The listing builds one solid part. Answer for the finished solid, in the listing's coordinates (mm). A direction names the side the tool comes from. Give positions to 0.01 mm unless a question says otherwise; leave off trailing zeros. Loops run counter-clockwise (first coordinate to the right, second up) from the corner with the lowest first, then second, coordinate; pieces in that order, holes last. Notation, with made-up numbers: (37.5, 54.5) - (49.5, 54.5) arc R13 cw to (49.5, 58.5) - close; hole circle Ø11 at (22.25, 63). An arc over 180 degrees is marked (long way). Write each question's results on one line, items separated by ' | '.
Autodesk Inventor part; units mm, degrees
ref_plane "YZ Plane" through (0, 0, 0) normal (1, 0, 0) x (0, 1, 0)
ref_plane "XZ Plane" through (0, 0, 0) normal (0, 1, 0) x (-1, 0, 0)
ref_plane "XY Plane" through (0, 0, 0) normal (0, 0, 1) x (1, 0, 0)
sketch "スケッチ1" plane through (0, 0, 0) normal (0, 0, 1) x (1, 0, 0)
  line L0 (-20, -10) -> (20, -10)
  line L1 (20, -10) -> (20, 10)
  line L2 (20, 10) -> (-20, 10)
  line L3 (-20, 10) -> (-20, -10)
  line L4 (-20, -10) -> (20, 10) construction
  line L5 (20, -10) -> (-20, 10) construction
  point P0 (0, 0)
  dimension "d0" = 40
  dimension "d1" = 20
extrude "押し出し1" add sketch "スケッチ1" along normal blind 3
sketch "スケッチ2" plane through (0, 0, 3) normal (0, 0, 1) x (1, 0, 0)
  line L0 (-16, -6) -> (16, -6) construction
  line L1 (16, -6) -> (16, 6) construction
  line L2 (16, 6) -> (-16, 6) construction
  line L3 (-16, 6) -> (-16, -6) construction
  line L4 (-16, -6) -> (16, 6) construction
  line L5 (16, -6) -> (-16, 6) construction
  point P0 (0, 0)
  dimension "d4" = 32
  dimension "d5" = 12
hole "穴1" at (-16, 6, 3) at (-16, -6, 3) at (16, -6, 3) at (16, 6, 3) direction (0, 0, -1) diameter 3.5 depth 8
sketch "スケッチ3" plane through (0, 0, 3) normal (0, 0, 1) x (1, 0, 0)
  circle A0 centre (-16, 6) radius 1.75
  line L0 (-16, 2.7668) -> (-18.8, 4.3834)
  line L1 (-18.8, 4.3834) -> (-18.8, 7.6166)
  line L2 (-18.8, 7.6166) -> (-16, 9.2332)
  line L3 (-16, 9.2332) -> (-13.2, 7.6166)
  line L4 (-13.2, 7.6166) -> (-13.2, 4.3834)
  line L5 (-13.2, 4.3834) -> (-16, 2.7668)
  point P0 (0, 0)
  point P1 (-21.5, 4.5639)
  point P2 (-21.5, 7.4361)
  dimension "d13" = 5.6
extrude "押し出し2" cut sketch "スケッチ3" against normal blind 2 contours A0 | L0 L1 L2 L3 L4 L5
pattern_linear "矩形状パターン1" count 2 spacing 32 along (1, 0, 0) count 2 spacing 12 along (0, -1, 0) of "押し出し2"
sketch "スケッチ4" plane through (-20, -10, 0) normal (0, -1, 0) x (1, 0, 0)
  line L0 (0, 3) -> (40, 3)
  line L1 (40, 3) -> (0, 3)
  line L2 (9.5, 3) -> (12.5, 6)
  line L3 (12.5, 6) -> (27.5, 6)
  line L4 (27.5, 6) -> (30.5, 3)
  line L5 (0, 0) -> (40, 0)
  point P0 (20, 0)
  point P1 (20, 6)
  point P2 (20, 0)
  dimension "d22" = 45
  dimension "d23" = 45
  dimension "d24" = 15
  dimension "d25" = 3
extrude "押し出し3" add sketch "スケッチ4" against normal up to surface (20 mm away)
fillet "フィレット1" radius 3 4 edges at (-20, 10, 1.5) (-20, -10, 1.5) (20, -10, 1.5) (20, 10, 1.5)
equation "\"d23\" = d22"
properties part number "3D_frame-connect-base1_3D プリント"
Item 1: A cutting plane is placed at D-D, the plane x = -15.5. Determine the outline of the cut face in (y, z), plus the area to 3 significant figures.
Values found:
outline: (-10, 0) - (-7.68, 0) - (-7.68, 1) - (-8.94, 1) - (-8.94, 3) - (-10, 3) - close; (-4.32, 0) - (4.32, 0) - (4.32, 1) - (3.06, 1) - (3.06, 3) - (-3.06, 3) - (-3.06, 1) - (-4.32, 1) - close; (7.68, 0) - (10, 0) - (10, 3) - (8.94, 3) - (8.94, 1) - (7.68, 1) - close | area: 29.7 mm²
Item 2: A cutting plane is placed at C-C, the plane y = -2. Determine the outline of the cut face in (x, z).
Values found:
outline: (-20, 0) - (20, 0) - (20, 3) - (10.5, 3) - (7.5, 6) - (-7.5, 6) - (-10.5, 3) - (-20, 3) - close
Item 3: For faces 1 (the face through (20, 0, 1)), 2 (the face through (14.7, -7.4, 1)), determine the directions among +Z, -Z, +X, -X, +Y, -Y from which every point of the face is accessible in a straight line to the end or side of a thin tool.
Values found:
face 1: +Z, -Z, +X, +Y, -Y | face 2: +Z
Item 4: Flat-ended cylindrical pins translate along their axes: P1, Ø4.5, axis at x = 15.5, y = 7, coming from the +Z side; P2, Ø4.5, axis at x = -16, y = 6, coming from the +Z side; P3, Ø3, axis at x = 16, y = 6, coming from the +Z side. Find the tip coordinate at first contact, or state that the pin passes through.
Values found:
P1: stops at z = 3 | P2: stops at z = 1 | P3: passes through
Item 5: Find the intervals of material crossed by line 1 along X through (y, z) = (6, 0.6); line 2 along Y through (x, z) = (16, 0.75); line 3 along Z through (x, y) = (-12.5, -4.25), in increasing order. Write a range as [from, to].
Values found:
line 1: x = [-20, -17.75], [-14.25, 14.25], [17.75, 20] | line 2: y = [-10, -7.75], [-4.25, 4.25], [7.75, 10] | line 3: z = [0, 3]
Item 6: A cutting plane is placed at A-A, the plane y = 6. Determine the outline of the cut face in (x, z), plus the area to 3 significant figures.
Values found:
outline: (-20, 0) - (-17.75, 0) - (-17.75, 1) - (-18.8, 1) - (-18.8, 3) - (-20, 3) - close; (-14.25, 0) - (14.25, 0) - (14.25, 1) - (13.2, 1) - (13.2, 3) - (10.5, 3) - (7.5, 6) - (-7.5, 6) - (-10.5, 3) - (-13.2, 3) - (-13.2, 1) - (-14.25, 1) - close; (17.75, 0) - (20, 0) - (20, 3) - (18.8, 3) - (18.8, 1) - (17.75, 1) - close | area: 145 mm²
Item 7: For a pull along Y with two mould halves and no side action, classify faces 3 (the face through (0, 0, 0)), 4 (the face through (-19.14, -9.1, 1.52)), 5 (the face through (-17.42, -3.586, 2.014)) as released by +Y, released by -Y, zero draft, split by the parting line, or undercut.
Values found:
face 3: zero draft | face 4: released by -Y | face 5: undercut
Item 8: A cutting plane is placed at B-B, the plane z = 1.7. Count the separate pieces of the cut face and the enclosed holes in it, plus the area to 3 significant figures.
Values found:
separate pieces: 1 | enclosed holes: 4 | area: 684 mm²
